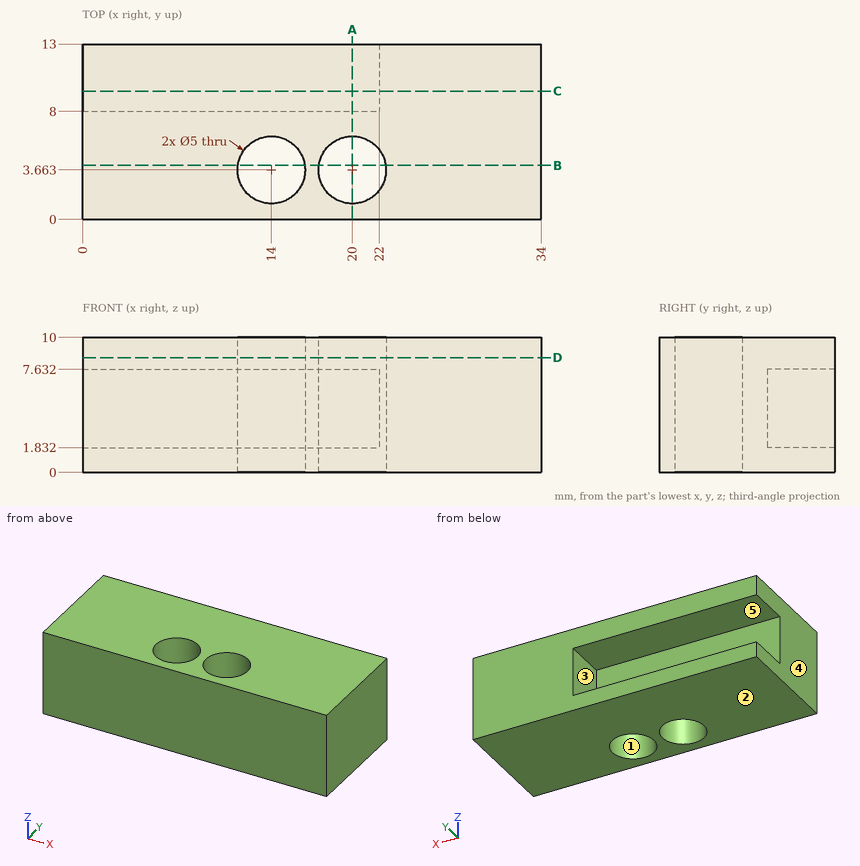
Verification items for this drawing (mm, ordinates from the low corner). A direction names the side the tool comes from. Round coordinates to 2 decimals unless told otherwise and drop trailing zeros. Order: outer loops, then holes, each group sorted by start corner. A loop starts at its lowest first (then second) coordinate and runs counter-clockwise, first axis right, second up. Notation, with made-up numbers: (56, 79.25) - (96, 79.25) arc R34 cw to (96, 112.25) - close; hole circle Ø2 at (11, 9). An arc over 180 degrees is marked (long way). Use CSV: the item, a comma, the result in double quotes.
(1) Section check D-D on z = 8.5. Record the boundary of the cut face in (x, y).
Entries:
outline,"(0, 0) - (34, 0) - (34, 13) - (0, 13) - close; hole circle Ø5 at (14, 3.66); hole circle Ø5 at (20, 3.66)"
(2) Section check A-A on x = 20. Record the boundary of the cut face in (y, z), and give its area (3 significant figures).
Entries:
outline,"(0, 0) - (1.16, 0) - (1.16, 10) - (0, 10) - close; (6.16, 0) - (13, 0) - (13, 1.83) - (8, 1.83) - (8, 7.63) - (13, 7.63) - (13, 10) - (6.16, 10) - close"
area,"51.0 mm^2"
(3) Section check B-B on y = 4. Record the boundary of the cut face in (x, z).
Entries:
outline,"(0, 0) - (11.52, 0) - (11.52, 10) - (0, 10) - close; (16.48, 0) - (17.52, 0) - (17.52, 10) - (16.48, 10) - close; (22.48, 0) - (34, 0) - (34, 10) - (22.48, 10) - close"
(4) Gauge pin test, flat end, axial feed: pin 1 Ø4.5 at (x, y) = (20, 3.66) entering from +Z. Record the tip position at first contact, or that the pin passes through.
Entries:
pin 1,"through"
(5) Thickness scan on probe 1 along X at (y, z) = (3.75, 2); probe 2 along Y at (x, z) = (14, 3); probe 3 along X at (y, z) = (3, 6.75). Record the ranges inside material, lowest first. Write a range as from..to.
Entries:
probe 1,"0..11.5, 16.5..17.5, 22.5..34"
probe 2,"0..1.16, 6.16..8"
probe 3,"0..11.59, 16.41..17.59, 22.41..34"
(6) Access from +Z, -Z, +X, -X, +Y, -Y to the whole of each face (thin tool, end or side, straight path). Record for the marked faces 4 and 5.
Entries:
face 4,"+Z, -Z, -X, +Y, -Y"
face 5,"-X, +Y"
(7) Mould release check, pull along Z, two halves, no side actions. Record for the marked faces 1, 2 and 3: released by +Z, released by -Z, zero draft, split by the parting line, or undercut.
Entries:
face 1,"zero draft"
face 2,"released by -Z"
face 3,"undercut"
(8) Section check C-C on y = 9.5. Record the boundary of the cut face in (x, z), and give its area (3 significant figures).
Entries:
outline,"(0, 0) - (34, 0) - (34, 10) - (0, 10) - (0, 7.63) - (22, 7.63) - (22, 1.83) - (0, 1.83) - close"
area,"212 mm^2"
